Geometry check sheet. Reference: the model listing, model coordinates, mm. A direction names the side the tool comes from. Round coordinates to 2 decimals unless told otherwise and drop trailing zeros. Write each loop counter-clockwise with the first axis right and the second up, starting at its lowest first coordinate (ties: lowest second). Pieces come first, ordered by that corner, then holes. Notation, with made-up numbers: M 69,84.5 L 114,84.5 A13 cw 114,108.5 Z; hole C -35.5,36 d3. An arc over 180 degrees is marked long. One line per item, written item: value. Start each with the question number.
1. Depth check by flat-ended pin: P1, Ø2, axis at x = -225.5, z = -558, coming from the -Y side; P2, Ø1, axis at y = 1.5, z = -461.5, coming from the +X side; P3, Ø7.5, axis at y = 29.5, z = -872, coming from the -X side. Enter the tip coordinate at first touch or a pass-through.
2. Section check A-A (y = 27.5). Record the boundary of the cut face in (x, z).
3. Section check B-B (z = -176). Record the boundary of the cut face in (x, y).
4. Access from +Z, -Z, +X, -X, +Y, -Y to the whole of each face (thin tool, end or side, straight path). Record for faces 5 (the flat face through (-202.415, -36, -15)), 6 (the flat face through (-195, -45.562, -15)), 7 (the flat face through (-199, -2, -860)), 8 (the flat face through (-202.415, 30, -15)).
5. Release check for a two-part mould opening along Z. For faces 1 (the flat face through (-195, 42.88, -15)), 2 (the flat face through (-217.415, -4, -439)), 3 (the flat face through (-224, -11, 0)), 4 (the flat face through (-199, -2, -30)) record: pulls with the +Z half, pulls with the -Z half, needs draft (parallel to the pull), parting line crosses it, or undercut.
6. Scan lines: probe 1 along Z at (x, y) = (-198.5, -18); probe 2 along X at (y, z) = (-12.5, -240); probe 3 along X at (y, z) = (10.5, -250). Record each from-to range of solid material in increasing order. Write a range as [from, to].
7. Section check D-D (x = -268). Record the boundary of the cut face in (y, z).
8. Section check C-C (y = -14). Record the boundary of the cut face in (x, z).
from build123d import *

# Parameters (mm, degrees)
BOSS_EXTRUDE1_DEPTH = 890
SKETCH4_W           = 830
SKETCH4_H           = 88.442264386
CUT_EXTRUDE1_DEPTH  = 30


with BuildPart() as part:
    # Sketch1 → Boss-Extrude1 (new body)
    with BuildSketch(Plane.XY):
        with BuildLine():
            ThreePointArc((-282.415201489, 0.868106525), (-253.025149144, 0.266679613), (-229.534634399, 17.939613952))
            Line((-229.534634399, 17.939613952), (-202.415201489, 17.939613952))
            Line((-202.415201489, 17.939613952), (-202.415201489, 42.879994244))
            Line((-202.415201489, 42.879994244), (-187.415201489, 42.879994244))
            Line((-187.415201489, 42.879994244), (-187.415201489, -45.562270142))
            Line((-187.415201489, -45.562270142), (-202.415201489, -45.562270142))
            Line((-202.415201489, -45.562270142), (-202.415201489, -25.562270142))
            Line((-202.415201489, -25.562270142), (-282.415201489, -25.562270142))
            Line((-282.415201489, -25.562270142), (-282.415201489, 0.868106525))
        make_face()
    extrude(amount=-BOSS_EXTRUDE1_DEPTH)

    # Sketch4 → Cut-Extrude1 (cut)
    with BuildSketch(Plane(origin=(-187.415201489, 0, 0), x_dir=(0, 0, -1), z_dir=(1, 0, 0))):
        with Locations((445, -1.341137949)):
            Rectangle(SKETCH4_W, SKETCH4_H)
    extrude(amount=-CUT_EXTRUDE1_DEPTH, mode=Mode.SUBTRACT)


solid = part.part
Result sheet:
1. P1: stops at y = -25.56
1. P2: stops at x = -217.42
1. P3: stops at x = -202.42
2. outline: M -202.42,-890 L -187.42,-890 L -187.42,-860 L -202.42,-860 Z; M -202.42,-30 L -187.42,-30 L -187.42,0 L -202.42,0 Z
3. outline: M -282.42,-25.56 L -217.42,-25.56 L -217.42,17.94 L -229.53,17.94 A45 cw -282.42,0.87 Z
4. face 5: +Z, -Z, -X, -Y
4. face 6: +Z, -Z, +X, -X, -Y
4. face 7: +X, +Y, -Y
4. face 8: +Z, -Z, -X, +Y
5. face 1: needs draft
5. face 2: undercut
5. face 3: pulls with the +Z half
5. face 4: undercut
6. probe 1: z = [-890, -860], [-30, 0]
6. probe 2: x = [-282.42, -217.42]
6. probe 3: x = [-235.82, -217.42]
7. outline: M -25.56,-890 L -1.89,-890 L -1.89,0 L -25.56,0 Z
8. outline: M -282.42,-890 L -187.42,-890 L -187.42,-860 L -217.42,-860 L -217.42,-30 L -187.42,-30 L -187.42,0 L -282.42,0 Z
